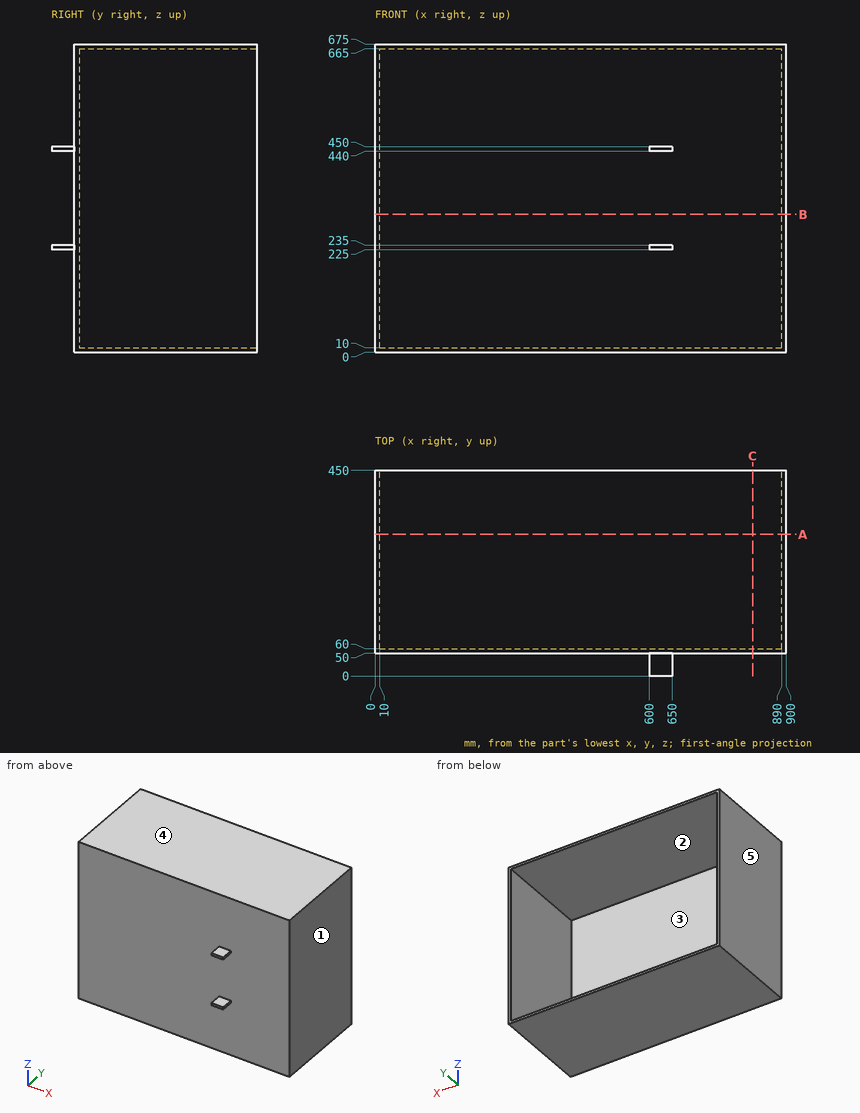
Geometry: see drawing. Coordinates: mm, zero at the bounding-box minimum. A direction names the side the tool comes from. Coordinates: 2 decimals unless noted, no trailing zeros. Loops run counter-clockwise (first coordinate to the right, second up) from the corner with the lowest first, then second, coordinate; pieces in that order, holes last. Notation, with made-up numbers: (-32.75, 22) - (13.25, 22) arc R17 ccw to (13.25, 30) - close; hole circle Ø5 at (32, 85.25). An arc over 180 degrees is marked (long way). Answer in a Markdown table with one row per item.
(1) Cut plane B-B on z = 302. Output: boundary loops of the cut face in (x, y), plus the area to 3 significant figures.
Model answer:
| item | result |
|---|---|
| outline | (0, 50) - (900, 50) - (900, 450) - (890, 450) - (890, 60) - (10, 60) - (10, 450) - (0, 450) - close |
| area | 16,800 mm² |
(2) Pin query (flat end, axial travel): P1, Ø5, axis at x = 326, z = 512, coming from the +Y side; P2, Ø5, axis at y = 31.5, z = 443, coming from the +X side; P3, Ø25, axis at x = 618, y = 35.5, coming from the -Z side. Return the tip coordinate at first contact, or that it passes through.
Model answer:
| item | result |
|---|---|
| P1 | stops at y = 60 |
| P2 | stops at x = 650 |
| P3 | stops at z = 225 |
(3) Mould query, pull axis Z, two halves, no side actions, for the marked faces 3, 4 and 5. Classes: pulls with the +Z half, pulls with the -Z half, needs draft (parallel to the pull), parting line crosses it, or undercut.
Model answer:
| item | result |
|---|---|
| face 3 | undercut |
| face 4 | pulls with the +Z half |
| face 5 | needs draft |
(4) Cut plane A-A on y = 310. Output: boundary loops of the cut face in (x, z).
Model answer:
| item | result |
|---|---|
| outline | (0, 0) - (900, 0) - (900, 675) - (0, 675) - close; hole (10, 10) - (890, 10) - (890, 665) - (10, 665) - close |
(5) Cut plane C-C on x = 826. Output: boundary loops of the cut face in (y, z), plus the area to 4 significant figures.
Model answer:
| item | result |
|---|---|
| outline | (50, 0) - (450, 0) - (450, 10) - (60, 10) - (60, 665) - (450, 665) - (450, 675) - (50, 675) - close |
| area | 14,550 mm² |
(6) Material intervals for L1, parallel to Z at x = 239.5, y = 72; L2, parallel to X at y = 304, z = 242; L3, parallel to Y at x = 638, z = 444.5, sorted ascending. Write a range as from..to.
Model answer:
| item | result |
|---|---|
| L1 | z = 0..10, 665..675 |
| L2 | x = 0..10, 890..900 |
| L3 | y = 0..60 |
(7) Set-up query: the marked faces 1 and 2. Return all of +Z, -Z, +X, -X, +Y, -Y with unobstructed straight access to the full face (end or side cutting, diameter ignored); none if empty.
Model answer:
| item | result |
|---|---|
| face 1 | +Z, -Z, +X, +Y, -Y |
| face 2 | +Y |
